Check sheet for the modelled part. Datum: model origin and axes. Units: mm. Face numbers are marked on the shaded views. A direction names the side the tool comes from. Give positions to 0.01 mm unless a question says otherwise; leave off trailing zeros. Order: outer loops, then holes, each group sorted by start corner. A loop starts at its lowest first (then second) coordinate and runs counter-clockwise, first axis right, second up. Notation, with made-up numbers: (-34, 52) -> (-22, 52) arc R14 ccw to (-22, 59) -> close; hole circle Ø1 at (-35, 76). An arc over 180 degrees is marked (long way). Answer in a Markdown table with one row per item. Add a question column.
(1) Go/stop test with a flat-tipped pin: pin 1 (1.2 mm diameter, centred on x = 52.5, y = 1.5, fed in from +Z). Record where the tip stops, or that it passes through.
(2) Cross-section at A-A (x = -5.5). Record the cut outline in (y, z).
(3) Cross-section at C-C (z = 7.5). Record the cut outline in (x, y), then the cut area to 3 significant figures.
(4) Cross-section at B-B (y = 9.5). Record the cut outline in (x, z), then the cut area to 3 significant figures.
(5) Thickness scan on L1, parallel to X at y = -17.5, z = 3.75; L2, parallel to Y at x = 26.5, z = 1; L3, parallel to X at y = -1, z = 1.75. Record the ranges inside material, lowest first. Write a range as [from, to].
(6) Set-up check for the marked faces 1 and 2: record each of +Z, -Z, +X, -X, +Y, -Y from which the full face is reachable in a straight line by a thin tool's end or side.
```python
from build123d import *

# Parameters (mm, degrees)
PAD002_DEPTH            = 56.5
BODY002_PLACEMENT_ANGLE = 90
PAD001_DEPTH            = 56.5
PAD_DEPTH               = 30
POCKET_DEPTH            = 28
POCKET001_DEPTH         = 2.001


with BuildPart() as corte_x:
    # Sketch004 → Pad002 (new body, symmetric)
    with BuildSketch(Plane.XZ):
        with BuildLine():
            Line((-58, 39.856555), (58, 39.856555))
            Line((58, 39.856555), (58, 9.856555))
            Line((58, 9.856555), (43, 9.856555))
            ThreePointArc((43, 9.856555), (38.129956, 8.810207), (34.119481, 5.855844))
            ThreePointArc((30, 4), (32.259108, 4.485378), (34.119481, 5.855844))
            Line((-30, 4), (30, 4))
            ThreePointArc((-34.119481, 5.855844), (-32.259108, 4.485378), (-30, 4))
            ThreePointArc((-34.119481, 5.855844), (-38.129956, 8.810207), (-43, 9.856555))
            Line((-58, 9.856555), (-43, 9.856555))
            Line((-58, 39.856555), (-58, 9.856555))
        make_face()
    extrude(amount=PAD002_DEPTH, both=True)


with BuildPart() as corte_x_1:
    # Body002 placement: moved
    add(corte_x.part.rotate(Axis((0, 0, 0), (0, 0, 1)), BODY002_PLACEMENT_ANGLE))


with BuildPart() as fusion:
    # Sketch003 → Pad001 (new body, symmetric)
    with BuildSketch(Plane.XZ):
        with BuildLine():
            Line((-58, 39.856555), (58, 39.856555))
            Line((58, 39.856555), (58, 9.856555))
            Line((58, 9.856555), (43, 9.856555))
            ThreePointArc((43, 9.856555), (38.129956, 8.810207), (34.119481, 5.855844))
            ThreePointArc((30, 4), (32.259108, 4.485378), (34.119481, 5.855844))
            Line((-30, 4), (30, 4))
            ThreePointArc((-34.119481, 5.855844), (-32.259108, 4.485378), (-30, 4))
            ThreePointArc((-34.119481, 5.855844), (-38.129956, 8.810207), (-43, 9.856555))
            Line((-58, 9.856555), (-43, 9.856555))
            Line((-58, 39.856555), (-58, 9.856555))
        make_face()
    extrude(amount=PAD001_DEPTH, both=True)

    # Fusion: union Corte X
    add(corte_x_1.part)


with BuildPart() as cut:
    # Sketch → Pad (new body)
    with BuildSketch(Plane.XY):
        with BuildLine():
            Line((-32, 54), (32, 54))
            ThreePointArc((54, 32), (47.556349, 47.556349), (32, 54))
            Line((54, 32), (54, -32))
            ThreePointArc((32, -54), (47.556349, -47.556349), (54, -32))
            Line((32, -54), (-32, -54))
            ThreePointArc((-54, -32), (-47.556349, -47.556349), (-32, -54))
            Line((-54, -32), (-54, 32))
            ThreePointArc((-32, 54), (-47.556349, 47.556349), (-54, 32))
        make_face()
    extrude(amount=PAD_DEPTH)

    # Sketch001 (on Face10 of Pad) → Pocket (cut)
    with BuildSketch(Plane.XY.offset(30)):
        with BuildLine():
            Line((-30, 50), (30, 50))
            ThreePointArc((50, 30), (44.142136, 44.142136), (30, 50))
            Line((50, 30), (50, -30))
            ThreePointArc((30, -50), (44.142136, -44.142136), (50, -30))
            Line((30, -50), (-30, -50))
            ThreePointArc((-50, -30), (-44.142136, -44.142136), (-30, -50))
            Line((-50, -30), (-50, 30))
            ThreePointArc((-30, 50), (-44.142136, 44.142136), (-50, 30))
        make_face()
    extrude(amount=-POCKET_DEPTH, mode=Mode.SUBTRACT)

    # Sketch002 (on Face19 of Pocket) → Pocket001 (cut, through all)
    with BuildSketch(Plane.XY.offset(2)):
        with BuildLine():
            Line((-29, 44.989147), (29, 44.989147))
            ThreePointArc((45, 28.989147), (40.313708, 40.302855), (29, 44.989147))
            Line((45, 28.989147), (45, -29))
            ThreePointArc((29, -45), (40.313708, -40.313708), (45, -29))
            Line((29, -45), (-29.589223, -45))
            ThreePointArc((-45.589223, -29), (-40.902931, -40.313708), (-29.589223, -45))
            Line((-45.589223, -29), (-45.589223, 29))
            ThreePointArc((-29, 44.989147), (-40.692655, 40.520147), (-45.589223, 29))
        make_face()
    extrude(amount=-POCKET001_DEPTH, mode=Mode.SUBTRACT)

    # Cut: cut Fusion
    add(fusion.part, mode=Mode.SUBTRACT)


solid = cut.part
```
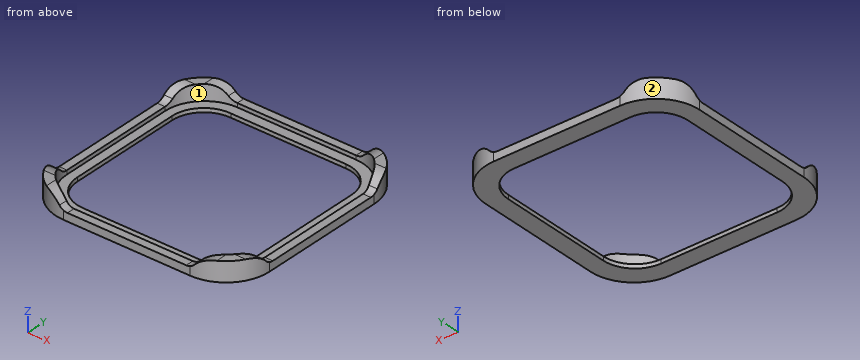
Answer below:
| question | item | result |
|---|---|---|
| 1 | pin 1 | stops at z = 4 |
| 2 | outline | (-54, 0) -> (-45, 0) -> (-45, 2) -> (-50, 2) -> (-50, 4) -> (-54, 4) -> close; (44.99, 0) -> (54, 0) -> (54, 4) -> (50, 4) -> (50, 2) -> (44.99, 2) -> close |
| 3 | outline | (-53.65, -35.91) arc R22 ccw to (-35.91, -53.65) -> (-35.91, -49.11) arc R20 cw to (-49.11, -35.91) -> close; (-53.65, 35.91) -> (-49.11, 35.91) arc R20 cw to (-35.91, 49.11) -> (-35.91, 53.65) arc R22 ccw to start; (35.91, -53.65) arc R22 ccw to (53.65, -35.91) -> (49.11, -35.91) arc R20 cw to (35.91, -49.11) -> close; (35.91, 49.11) arc R20 cw to (49.11, 35.91) -> (53.65, 35.91) arc R22 ccw to (35.91, 53.65) -> close |
| 3 | area | 433 mm² |
| 4 | outline | (-54, 0) -> (-45.59, 0) -> (-45.59, 2) -> (-50, 2) -> (-50, 4) -> (-54, 4) -> close; (45, 0) -> (54, 0) -> (54, 4) -> (50, 4) -> (50, 2) -> (45, 2) -> close |
| 4 | area | 50.8 mm² |
| 5 | L1 | x = [-54, -50], [50, 54] |
| 5 | L2 | y = [-54, -45], [44.99, 54] |
| 5 | L3 | x = [-54, -45.59], [45, 54] |
| 6 | face 1 | +Z |
| 6 | face 2 | +Z, -Z, -X, +Y |
